Can you work these out from the model? Positions are in its coordinate system, mm. A direction names the side the tool comes from. Give positions to 0.01 mm unless a question says otherwise; leave off trailing zeros. Order: outer loops, then holes, each group sorted by start corner. A loop starts at its lowest first (then second) coordinate and runs counter-clockwise, first axis right, second up. Notation, with made-up numbers: (67.5, 5) -> (98.5, 5) arc R24 ccw to (98.5, 19) -> close; hole circle Ø10 at (53, 9.25). An arc over 180 degrees is marked (long way). Answer as a JSON object with one key per item and string values.
```python
from build123d import *

# Parameters (mm, degrees)
SKETCH005_R              = 43.25
PAD002_DEPTH             = 18
SKETCH006_R              = 33.25
SKETCH006_R_2            = 28.25
POCKET003_DEPTH          = 10
HOLE_D                   = 5
HOLE_CBORE_D             = 11
HOLE_CBORE_DEPTH         = 10
SKETCH008_W              = 40
SKETCH008_H              = 40
SKETCH008_R              = 10
POCKET004_DEPTH          = 1
CLONE003_PLACEMENT_ANGLE = 180


with BuildPart() as part:
    # Sketch005 → Pad002 (new body)
    with BuildSketch(Plane.XY):
        Circle(SKETCH005_R)
    extrude(amount=PAD002_DEPTH)

    # Sketch006 (on Face3 of Pad002) → Pocket003 (cut)
    with BuildSketch(Plane.XY.offset(18)):
        Circle(SKETCH006_R)
        Circle(SKETCH006_R_2, mode=Mode.SUBTRACT)
    extrude(amount=-POCKET003_DEPTH, mode=Mode.SUBTRACT)

    # Hole (through all)
    with Locations(Plane.XY.offset(18)):
        with Locations((0, 0)):
            CounterBoreHole(HOLE_D / 2, HOLE_CBORE_D / 2, HOLE_CBORE_DEPTH)

    # Sketch008 (on Face2 of Hole) → Pocket004 (cut)
    with BuildSketch(Plane(origin=(0, 0, 0), x_dir=(1, 0, 0), z_dir=(0, 0, -1))):
        Rectangle(SKETCH008_W, SKETCH008_H)
        Circle(SKETCH008_R, mode=Mode.SUBTRACT)
    extrude(amount=-POCKET004_DEPTH, mode=Mode.SUBTRACT)


with BuildPart() as part_1:
    # Clone003 placement: moved
    add(part.part.moved(Location((0, 0, 18))).rotate(Axis((0, 0, 18), (1, 0, 0)), CLONE003_PLACEMENT_ANGLE))


solid = part_1.part
```
1. For faces 1 (the face through (15.19, -23.82, 4.93)), 2 (the face through (-10, 32, 0)), which set-ups out of +Z, -Z, +X, -X, +Y, -Y let a thin tool reach every point of the face, with its end or its side?
Worked answers:
{"face 1": "-Z", "face 2": "-Z, +X, -X, +Y, -Y"}
2. If we mould it in two halves opening along Y, with no side actions, what happens to faces 3 (the face through (-2.17, -9.76, 17.51)), 4 (the face through (-5, 9, 17)), 5 (the face through (28, -1, 18)), 6 (the face through (-34.32, 26.32, 9.13))? For each: +Y half, -Y half, draft (parallel to the pull), parting line (faces both ways), or undercut.
Worked answers:
{"face 3": "undercut", "face 4": "undercut", "face 5": "draft", "face 6": "parting line"}
3. Please list where these lines run through material, in increasing order: L1, parallel to Y at x = 0, z = 5.25; L2, parallel to Y at x = 0, z = 13.
Worked answers:
{"L1": "-43.25 to -33.25, -28.25 to -5.5, 5.5 to 28.25, 33.25 to 43.25", "L2": "-43.25 to -2.5, 2.5 to 43.25"}
4. If we section it at D-D on x = 11.5: Please give me the cut outline in (y, z), then the cut area to 3 significant figures.
Worked answers:
{"outline": "(-41.69, 0) -> (-31.2, 0) -> (-31.2, 10) -> (-25.8, 10) -> (-25.8, 0) -> (25.8, 0) -> (25.8, 10) -> (31.2, 10) -> (31.2, 0) -> (41.69, 0) -> (41.69, 18) -> (20, 18) -> (20, 17) -> (-20, 17) -> (-20, 18) -> (-41.69, 18) -> close", "area": "1,350 mm²"}
5. Will these pins go through, and if not, where does the flat tip stop? pin 1 Ø1 at (x, z) = (11.5, 15.5) entering from -Y; pin 2 Ø0.8 at (x, z) = (-6, 17.5) entering from +Y; pin 3 Ø10 at (x, z) = (15, 6) entering from +Y.
Worked answers:
{"pin 1": "y = -41.83", "pin 2": "y = 42.89", "pin 3": "y = 42.08"}
6. If we section it at C-C on z = 5.25: Please give me the cut outline in (x, y).
Worked answers:
{"outline": "circle Ø86.5 at (0, 0); circle Ø56.5 at (0, 0); hole circle Ø66.5 at (0, 0); hole circle Ø11 at (0, 0)"}
7. If we section it at A-A on y = 0: Please give me the cut outline in (x, z), then the cut area to 3 significant figures.
Worked answers:
{"outline": "(-43.25, 0) -> (-33.25, 0) -> (-33.25, 10) -> (-28.25, 10) -> (-28.25, 0) -> (-5.5, 0) -> (-5.5, 10) -> (-2.5, 10) -> (-2.5, 18) -> (-10, 18) -> (-10, 17) -> (-20, 17) -> (-20, 18) -> (-43.25, 18) -> close; (2.5, 10) -> (5.5, 10) -> (5.5, 0) -> (28.25, 0) -> (28.25, 10) -> (33.25, 10) -> (33.25, 0) -> (43.25, 0) -> (43.25, 18) -> (20, 18) -> (20, 17) -> (10, 17) -> (10, 18) -> (2.5, 18) -> close", "area": "1,290 mm²"}
